The listing builds one solid part. Answer for the finished solid, in the listing's coordinates (mm). Face numbers are marked on the shaded views. Round coordinates to 2 decimals unless told otherwise and drop trailing zeros. Order: outer loops, then holes, each group sorted by start corner. A loop starts at its lowest first (then second) coordinate and runs counter-clockwise, first axis right, second up. Notation, with made-up numbers: (-9, 45) - (12, 45) arc R17 cw to (12, 55) - close; hole circle Ø7 at (49.25, 79). An arc over 180 degrees is marked (long way). Write item = value, one per line.
from build123d import *

# Parameters (mm, degrees)
SKIZZE1_W                                            = 40
SKIZZE1_H                                            = 40
AUFSATZ_LINEAR_AUSTRAGEN1_DEPTH                      = 15
SKIZZE3_R                                            = 7.5
SCHNITT_LINEAR_AUSTRAGEN1_DEPTH                      = 12
DURCHGANGSLOCH_F_R_M41_D                             = 4.5
DURCHGANGSLOCH_F_R_M1_61_D                           = 1.8
FORMSENKUNG_F_R_M1_6_SENKSCHRAUBE_MIT_SC_D           = 1.8
FORMSENKUNG_F_R_M1_6_SENKSCHRAUBE_MIT_SC_CSINK_D     = 3.6
FORMSENKUNG_F_R_M1_6_SENKSCHRAUBE_MIT_SC_CSINK_ANGLE = 90


with BuildPart() as part:
    # Skizze1 → Aufsatz-Linear austragen1 (new body)
    with BuildSketch(Plane.XY):
        with Locations((4.479166667, 4.375)):
            Rectangle(SKIZZE1_W, SKIZZE1_H)
    extrude(amount=AUFSATZ_LINEAR_AUSTRAGEN1_DEPTH)

    # Skizze3 → Schnitt-Linear austragen1 (cut)
    with BuildSketch(Plane.XY.offset(15)):
        with Locations((4.479166667, 4.375)):
            Circle(SKIZZE3_R)
    extrude(amount=-SCHNITT_LINEAR_AUSTRAGEN1_DEPTH, mode=Mode.SUBTRACT)

    # Durchgangsloch für M41 (through all)
    with Locations(Plane.XY.offset(3)):
        with Locations((4.479166667, 4.375)):
            Hole(DURCHGANGSLOCH_F_R_M41_D / 2)

    # Durchgangsloch für M1.61 (through all)
    with Locations(Plane.XY.offset(3)):
        with Locations((4.479166667, 8.875), (4.479166667, -0.125)):
            Hole(DURCHGANGSLOCH_F_R_M1_61_D / 2)

    # Formsenkung für M1.6 Senkschraube mit Schlitz/Kreuzschlitz1 (through all)
    with Locations(Plane(origin=(0, 0, 0), x_dir=(-1, 0, 0), z_dir=(0, 0, -1))):
        with Locations((-19.979166667, 19.875), (11.020833333, 19.875), (11.020833333, -11.125), (-19.979166667, -11.125)):
            CounterSinkHole(FORMSENKUNG_F_R_M1_6_SENKSCHRAUBE_MIT_SC_D / 2, FORMSENKUNG_F_R_M1_6_SENKSCHRAUBE_MIT_SC_CSINK_D / 2, counter_sink_angle=FORMSENKUNG_F_R_M1_6_SENKSCHRAUBE_MIT_SC_CSINK_ANGLE)


solid = part.part
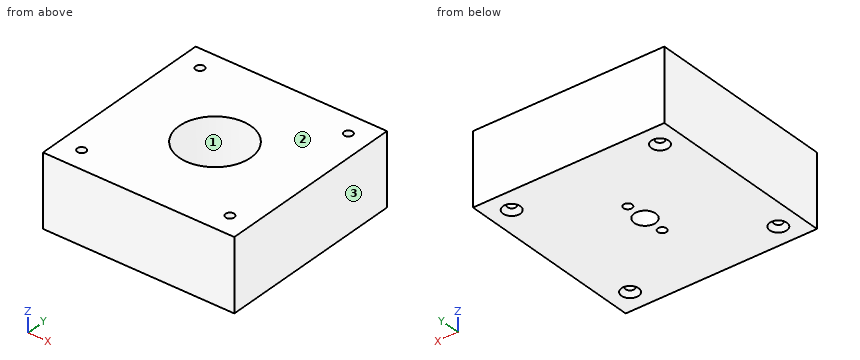
Q1. Section D-D on y = -2.5 is taken. Determine the outline of the cut face in (x, z).
Model answer:
outline = (-15.52, 0) - (24.48, 0) - (24.48, 15) - (7.48, 15) - (7.48, 3) - (1.48, 3) - (1.48, 15) - (-15.52, 15) - close
Q2. Section C-C on z = 5.75 is taken. Determine the outline of the cut face in (x, y) (3 decimals), then the cut area to 3 significant figures.
Model answer:
outline = (-15.521, -15.625) - (24.479, -15.625) - (24.479, 24.375) - (-15.521, 24.375) - close; hole circle Ø1.8 at (-11.021, -11.125); hole circle Ø1.8 at (-11.021, 19.875); hole circle Ø15 at (4.479, 4.375); hole circle Ø1.8 at (19.979, -11.125); hole circle Ø1.8 at (19.979, 19.875)
area = 1,410 mm^2
Q3. Section B-B on x = -2 is taken. Determine the outline of the cut face in (y, z) (3 decimals), then the cut area to 3 significant figures.
Model answer:
outline = (-15.625, 0) - (24.375, 0) - (24.375, 15) - (8.153, 15) - (8.153, 3) - (0.597, 3) - (0.597, 15) - (-15.625, 15) - close
area = 509 mm^2
Q4. Section A-A on z = 1.75 is taken. Determine the outline of the cut face in (x, y) (3 decimals), then the cut area to 3 significant figures.
Model answer:
outline = (-15.521, -15.625) - (24.479, -15.625) - (24.479, 24.375) - (-15.521, 24.375) - close; hole circle Ø1.8 at (-11.021, -11.125); hole circle Ø1.8 at (-11.021, 19.875); hole circle Ø4.5 at (4.479, 4.375); hole circle Ø1.8 at (4.479, -0.125); hole circle Ø1.8 at (4.479, 8.875); hole circle Ø1.8 at (19.979, -11.125); hole circle Ø1.8 at (19.979, 19.875)
area = 1,570 mm^2
Q5. Determine the mould class of the marked faces 1, 2 and 3 for opening direction X: released by +X, released by -X, zero draft, split by the parting line, or undercut.
Model answer:
face_1 = undercut
face_2 = zero draft
face_3 = released by +X
Q6. Flat-ended cylindrical pins translate along their axes: P1, Ø4.5, axis at x = 7, y = 3.5, coming from the +Z side; P2, Ø17, axis at x = 4.48, y = 4.38, coming from the -Z side; P3, Ø2, axis at x = 19.98, y = 19.88, coming from the -Z side. Find the tip coordinate at first contact, or state that the pin passes through.
Model answer:
P1 = 3
P2 = 0
P3 = 0.79
Q7. Find the intervals of material crossed by line 1 (Y direction, x = -10.5, z = 2) (3 decimals); line 2 (Y direction, x = 7, z = 8.5) (3 decimals); line 3 (Z direction, x = 0.5, y = 5), in increasing order. Write a range as from..to.
Model answer:
line_1 = -15.625..-11.859, -10.391..19.141, 20.609..24.375
line_2 = -15.625..-2.689, 11.439..24.375
line_3 = 0..3
